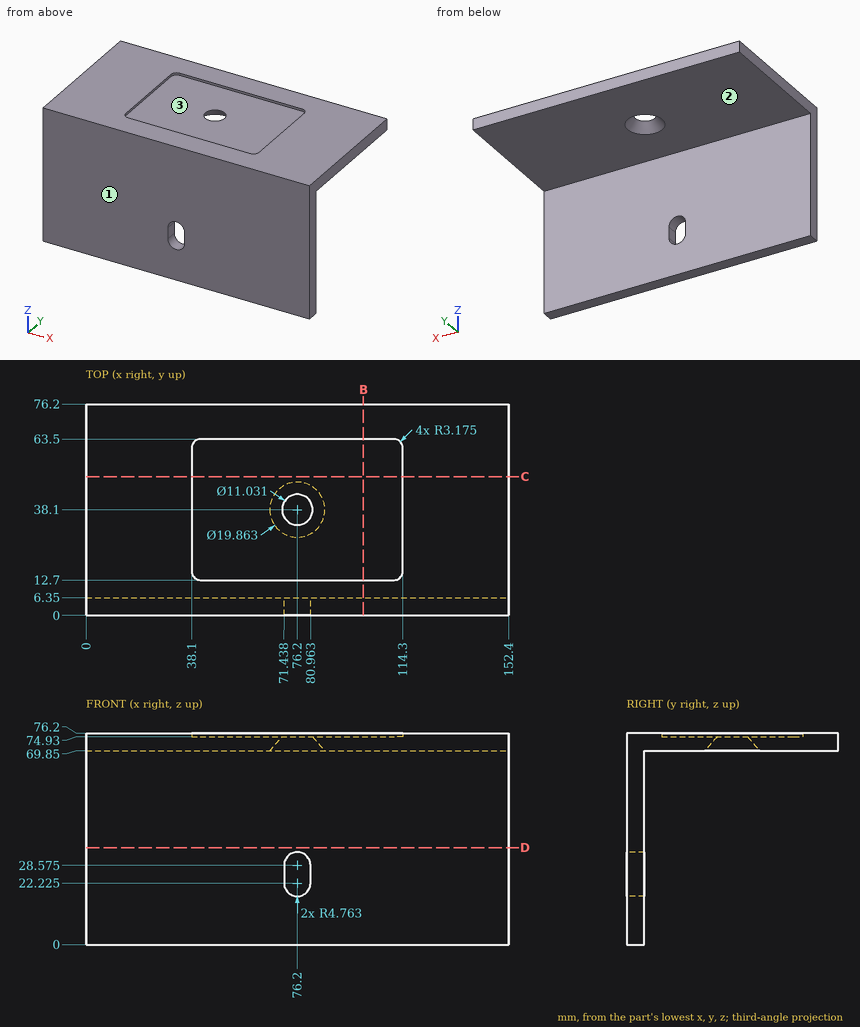
The figure shows three views and two pictorial views of one solid part (mm, origin at its lowest corner). Answer the questions. A direction names the side the tool comes from. Round coordinates to 2 decimals unless told otherwise and drop trailing zeros. Write each loop counter-clockwise with the first axis right and the second up, starting at its lowest first coordinate (ties: lowest second). Pieces come first, ordered by that corner, then holes. Notation, with made-up numbers: (-1.5, 45) -> (26.5, 45) arc R32 cw to (26.5, 75) -> close; hole circle Ø7 at (4.25, -30). An arc over 180 degrees is marked (long way). Write each question's results on one line, items separated by ' | '.
Q1. Section B-B, the plane x = 100 is taken. Write down the section's boundary in (y, z).
Data:
outline: (0, 0) -> (6.35, 0) -> (6.35, 69.85) -> (76.2, 69.85) -> (76.2, 76.2) -> (63.5, 76.2) -> (63.5, 74.93) -> (12.7, 74.93) -> (12.7, 76.2) -> (0, 76.2) -> close
Q2. Section D-D, the plane z = 35 is taken. Write down the section's boundary in (x, y).
Data:
outline: (0, 0) -> (152.4, 0) -> (152.4, 6.35) -> (0, 6.35) -> close
Q3. Which of the six approach directions +Z, -Z, +X, -X, +Y, -Y give full straight-line access (tool end or side, diameter ignored) to the marked faces 1, 2 and 3?
Data:
face 1: +Z, -Z, +X, -X, -Y | face 2: -Z, +X, -X, +Y | face 3: +Z
Q4. Section C-C, the plane y = 50 is taken. Write down the section's boundary in (x, z), then the cut area to 3 significant figures.
Data:
outline: (0, 69.85) -> (152.4, 69.85) -> (152.4, 76.2) -> (114.3, 76.2) -> (114.3, 74.93) -> (38.1, 74.93) -> (38.1, 76.2) -> (0, 76.2) -> close | area: 871 mm^2
Q5. Flat-ended cylindrical pins translate along their axes: P1, Ø6, axis at x = 41.5, y = 28.5, coming from the -Z side; P2, Ø21, axis at x = 48, z = 26.5, coming from the +Y side. Find the tip coordinate at first contact, or state that the pin passes through.
Data:
P1: z = 69.85 | P2: y = 6.35
Q6. Straight lines are drawn through the part: line 1 along Y through (x, z) = (87, 17); line 2 along Z through (x, y) = (38.5, 47.5); line 3 along Z through (x, y) = (27, 9). For each, find the intervals that lie inside material, in ascending order. Write a range as [from, to].
Data:
line 1: [0, 6.35] | line 2: [69.85, 74.93] | line 3: [69.85, 76.2]
